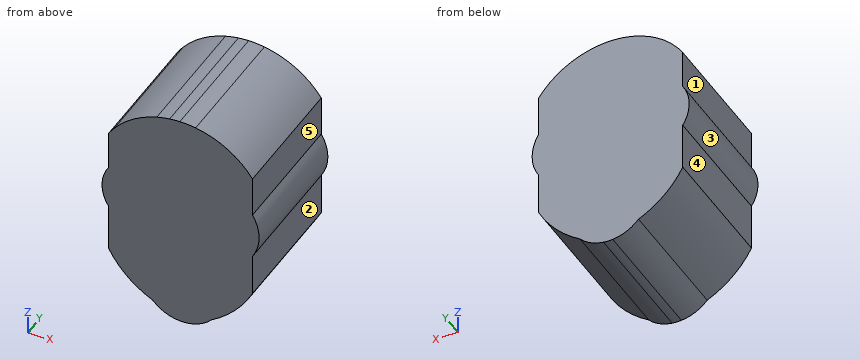
```python
from build123d import *

# Parameters (mm, degrees)
F0_R     = 2.5545771164
F1_DEPTH = 25.4


with BuildPart() as f1:
    # F0 (on Front) → F1 (new body)
    with BuildSketch(Plane.XZ):
        with BuildLine():
            ThreePointArc((5.5173615, -12.2159869029), (10.1722749208, -8.349582263), (13.5962825941, -3.3602461101))
            Line((13.5962825941, -3.3602461101), (13.5962825941, 4.8974110327))
            Line((13.5962825941, 4.8974110327), (13.5962825941, 14.0348058194))
            Line((13.5962825941, 14.0348058194), (13.5962825941, 22.0215348944))
            ThreePointArc((13.5962825941, 22.0215348944), (7.0004948303, 23.9860138876), (2.4660649804, 29.163130834))
            ThreePointArc((2.4660649804, 29.163130834), (0.9278228298, 29.3509775836), (-0.6211690061, 29.3967990577))
            ThreePointArc((-0.6211690061, 29.3967990577), (-6.7674815186, 23.985159586), (-14.5891272378, 21.5592870597))
            Line((-14.5891272378, 21.5592870597), (-14.5891272378, 14.0348058194))
            Line((-14.5891272378, 14.0348058194), (-14.5891272378, 5.4543889128))
            Line((-14.5891272378, 5.4543889128), (-14.5891272378, -3.8224939448))
            ThreePointArc((-14.5891272378, -3.8224939448), (-10.9382332049, -8.6804949763), (-5.9286805309, -12.1204925444))
            ThreePointArc((-5.9286805309, -12.1204925444), (-3.6496885116, -13.8889948714), (-0.8791223551, -14.6923430381))
            Line((-0.8791223551, -14.6923430381), (-1.524235704, -12.442663312))
            Line((-1.524235704, -12.442663312), (-0.8053276106, -12.442663312))
            Line((-0.8053276106, -12.442663312), (1.6964728711, -12.442663312))
            Line((1.6964728711, -12.442663312), (0.9172699194, -14.6494874696))
            ThreePointArc((0.9172699194, -14.6494874696), (3.4296394179, -13.8340966584), (5.5173615, -12.2159869029))
        make_face()
        with BuildLine():
            ThreePointArc((4.1042999377, -5.4248327223), (-0.1629000623, -7.0430521679), (-4.4301000623, -5.4248327223))
            ThreePointArc((-4.4301000623, -5.4248327223), (-0.1629000623, -4.7424848144), (4.1042999377, -5.4248327223))
        make_face(mode=Mode.SUBTRACT)
        with BuildLine():
            ThreePointArc((-5.5468901992, -5.0085484982), (-0.1374995827, -3.3742803628), (5.2100941539, -5.2006375045))
            ThreePointArc((5.2100941539, -5.2006375045), (-0.1549943991, -4.3539900851), (-5.5468901992, -5.0085484982))
        make_face(mode=Mode.SUBTRACT)
        with BuildLine():
            Line((-1.1811126024, 3.6468864419), (0, 8.5498616099))
            Line((0, 8.5498616099), (0.9875110118, 3.6468864419))
            ThreePointArc((0.9875110118, 3.6468864419), (-0.0968007953, 3.4477826759), (-1.1811126024, 3.6468864419))
        make_face(mode=Mode.SUBTRACT)
        with Locations((-5.9286805309, 12.5275942676)):
            Circle(F0_R, mode=Mode.SUBTRACT)
        with Locations((5.2393031111, 12.5385038482)):
            Circle(F0_R, mode=Mode.SUBTRACT)
        with Locations((-5.9286805309, 12.5275942676)):
            Circle(F0_R)
        with Locations((5.2393031111, 12.5385038482)):
            Circle(F0_R)
        with BuildLine():
            ThreePointArc((-14.5891272378, 21.5592870597), (-8.0233624944, 24.4917266981), (-2.6266052104, 29.2439345762))
            ThreePointArc((-2.6266052104, 29.2439345762), (-3.8995230158, 29.0200605642), (-5.1515523835, 28.6993398522))
            ThreePointArc((-5.1515523835, 28.6993398522), (-9.00952741, 25.5027604596), (-13.4385656433, 23.1606008906))
            ThreePointArc((-13.4385656433, 23.1606008906), (-14.0372751917, 22.3767777904), (-14.5891272378, 21.5592870597))
        make_face()
        with BuildLine():
            ThreePointArc((-14.5891272378, 21.5592870597), (-6.7674815186, 23.985159586), (-0.6211690061, 29.3967990577))
            ThreePointArc((-0.6211690061, 29.3967990577), (-1.6261684912, 29.3502963848), (-2.6266052104, 29.2439345762))
            ThreePointArc((-2.6266052104, 29.2439345762), (-8.0233624944, 24.4917266981), (-14.5891272378, 21.5592870597))
        make_face()
        with BuildLine():
            ThreePointArc((4.1042999377, -5.4248327223), (-0.1629000623, -4.7424848144), (-4.4301000623, -5.4248327223))
            ThreePointArc((-4.4301000623, -5.4248327223), (-0.1629000623, -7.0430521679), (4.1042999377, -5.4248327223))
        make_face()
        with BuildLine():
            ThreePointArc((2.4660649804, 29.163130834), (8.0510188895, 25.6232615682), (13.5962825941, 22.0215348944))
            ThreePointArc((13.5962825941, 22.0215348944), (8.7605664052, 26.7290953796), (2.4660649804, 29.163130834))
        make_face()
        with BuildLine():
            ThreePointArc((2.4660649804, 29.163130834), (7.5150761888, 24.7879918416), (13.5962825941, 22.0215348944))
            ThreePointArc((13.5962825941, 22.0215348944), (8.0510188895, 25.6232615682), (2.4660649804, 29.163130834))
        make_face()
        with BuildLine():
            ThreePointArc((2.4660649804, 29.163130834), (7.0004948303, 23.9860138876), (13.5962825941, 22.0215348944))
            ThreePointArc((13.5962825941, 22.0215348944), (7.5150761888, 24.7879918416), (2.4660649804, 29.163130834))
        make_face()
        with BuildLine():
            ThreePointArc((-13.4385656433, 23.1606008906), (-9.00952741, 25.5027604596), (-5.1515523835, 28.6993398522))
            ThreePointArc((-5.1515523835, 28.6993398522), (-9.7137087169, 26.5563504315), (-13.4385656433, 23.1606008906))
        make_face()
        with BuildLine():
            Line((13.5962825941, 14.0348058194), (13.5962825941, 4.8974110327))
            ThreePointArc((13.5962825941, 4.8974110327), (14.8954022083, 9.4661084261), (13.5962825941, 14.0348058194))
        make_face()
        with BuildLine():
            ThreePointArc((-14.5891272378, 14.0348058194), (-15.8586854832, 9.7445973661), (-14.5891272378, 5.4543889128))
            Line((-14.5891272378, 5.4543889128), (-14.5891272378, 14.0348058194))
        make_face()
        with BuildLine():
            ThreePointArc((-5.5468901992, -5.0085484982), (-0.1549943991, -4.3539900851), (5.2100941539, -5.2006375045))
            ThreePointArc((5.2100941539, -5.2006375045), (-0.1374995827, -3.3742803628), (-5.5468901992, -5.0085484982))
        make_face()
        with BuildLine():
            Line((0.9875110118, 3.6468864419), (0, 8.5498616099))
            Line((0, 8.5498616099), (-1.1811126024, 3.6468864419))
            ThreePointArc((-1.1811126024, 3.6468864419), (-0.0968007953, 3.4477826759), (0.9875110118, 3.6468864419))
        make_face()
        Polygon((-0.8791223551, -14.6923430381), (0.9172699194, -14.6494874696), (1.6964728711, -12.442663312), (-0.8053276106, -12.442663312), (-1.524235704, -12.442663312), align=None)
        with BuildLine():
            ThreePointArc((-0.8791223551, -14.6923430381), (0.0203310213, -14.7236153998), (0.9172699194, -14.6494874696))
            Line((0.9172699194, -14.6494874696), (-0.8791223551, -14.6923430381))
        make_face()
    extrude(amount=F1_DEPTH)


solid = f1.part
```
Part model, mm, in its own coordinate system. Face numbers are marked on the shaded views. A direction names the side the tool comes from. Round coordinates to 2 decimals unless told otherwise and drop trailing zeros. Loops run counter-clockwise (first coordinate to the right, second up) from the corner with the lowest first, then second, coordinate; pieces in that order, holes last.
1. Slice it at B-B (z = 18). Give the cut face in (x, y), and give its area (3 significant figures).
Solutions:
outline: (-14.59, -25.4) - (13.6, -25.4) - (13.6, 0) - (-14.59, 0) - close
area: 716 mm2
2. Drill centre lines: line 1 along X through (y, z) = (-23, 21.5); line 2 along Z through (x, y) = (-5.5, -4.5); line 3 along X through (y, z) = (-17, 12.5). Where is each one in solid material? Low to high.
Solutions:
line 1: x = -14.59 to 13.6
line 2: z = -12.57 to 28.59
line 3: x = -15.36 to 14.35
3. 3-axis set-ups, long thin cutter, end or side, ignore diameter. For the marked faces 1, 2, 3, 4 and 5: which of +Z, -Z, +X, -X, +Y, -Y reach the whole face in a straight line?
Solutions:
face 1: +Z, -X, +Y, -Y
face 2: -Z, +X, +Y, -Y
face 3: -X, +Y, -Y
face 4: -Z, -X, +Y, -Y
face 5: +Z, +X, +Y, -Y
4. Slice it at A-A (y = -8.5). Give the cut face in (x, z).
Solutions:
outline: (-14.59, -3.82) arc R18.8 ccw to (-5.93, -12.12) arc R7.68 ccw to (5.52, -12.22) arc R21.98 ccw to (13.6, -3.36) - (13.6, 4.9) arc R8.68 ccw to (13.6, 14.03) - (13.6, 22.02) arc R16.86 ccw to (-14.59, 21.56) - (-14.59, 14.03) arc R7.88 ccw to (-14.59, 5.45) - close
5. Slice it at C-C (x = 10.5). Give the cut face in (y, z).
Solutions:
outline: (-25.4, -7.98) - (0, -7.98) - (0, 25.45) - (-25.4, 25.45) - close
6. Flat gauge pins, fed straight in: pin 1 (4 mm diameter, centred on y = -7, z = 22.5, fed in from +X); pin 2 (1 mm diameter, centred on y = -6, z = 13.5, fed in from +X); pin 3 (4 mm diameter, centred on x = 8.5, y = -13, fed in from +Z); pin 4 (5 mm diameter, centred on x = -5.5, z = 21.5, fed in from +Y). Where does each tip first touch, or does it go through?
Solutions:
pin 1: stops at x = 13.6
pin 2: stops at x = 14.14
pin 3: stops at z = 27.95
pin 4: stops at y = 0
